from build123d import *

# Parameters (mm, degrees)
F1_DEPTH      = 12.7
F1_DEPTH_BACK = 12.7
F0_W          = 371.475
F0_H          = 622.3
F2_DEPTH      = 9.398
F2_DEPTH_BACK = 9.398
F3_W          = 371.475
F3_H          = 12.7
F4_DEPTH      = 12.7


# Not quite as in the source:
# - a feature names something its author has since deleted; it is built from what else it names


with BuildPart() as f1:
    # F0 (on Front) → F1 (new body, two sides)
    with BuildSketch(Plane.XZ) as f1_sk:
        Polygon((263.0418609804, 506.0493900317), (634.5168609804, 506.0493900317), (653.5668609804, 525.0993900317), (243.9918609804, 525.0993900317), align=None)
        Polygon((653.5668609804, 525.0993900317), (634.5168609804, 506.0493900317), (634.5168609804, -116.2506099683), (653.5668609804, -135.3006099683), align=None)
        Polygon((653.5668609804, -135.3006099683), (634.5168609804, -116.2506099683), (263.0418609804, -116.2506099683), (243.9918609804, -135.3006099683), align=None)
        Polygon((263.0418609804, -116.2506099683), (263.0418609804, 506.0493900317), (243.9918609804, 525.0993900317), (243.9918609804, -135.3006099683), align=None)
    extrude(amount=-F1_DEPTH)
    extrude(f1_sk.sketch, amount=F1_DEPTH_BACK)

    # F0 (on Front) → F2 (join, two sides)
    with BuildSketch(Plane.XZ) as f2_sk:
        Polygon((653.5668609804, 525.0993900317), (634.5168609804, 506.0493900317), (634.5168609804, -116.2506099683), (653.5668609804, -135.3006099683), align=None)
        Polygon((263.0418609804, 506.0493900317), (634.5168609804, 506.0493900317), (653.5668609804, 525.0993900317), (243.9918609804, 525.0993900317), align=None)
        Polygon((653.5668609804, -135.3006099683), (634.5168609804, -116.2506099683), (263.0418609804, -116.2506099683), (243.9918609804, -135.3006099683), align=None)
        with Locations((448.7793609804, 194.8993900317)):
            Rectangle(F0_W, F0_H)
        Polygon((263.0418609804, -116.2506099683), (263.0418609804, 506.0493900317), (243.9918609804, 525.0993900317), (243.9918609804, -135.3006099683), align=None)
    extrude(amount=-F2_DEPTH)
    extrude(f2_sk.sketch, amount=F2_DEPTH_BACK)

    # F3 (on face) → F4 (cut)
    with BuildSketch(Plane.XZ):
        Polygon((455.1293609804, 105.9993900317), (455.1293609804, 384.1293900317), (634.5168609804, 384.1293900317), (634.5168609804, 396.8293900317), (263.0418609804, 396.8293900317), (263.0418609804, 384.1293900317), (442.4293609804, 384.1293900317), (442.4293609804, 105.9993900317), (263.0418609804, 105.9993900317), (263.0418609804, 93.2993900317), (634.5168609804, 93.2993900317), (634.5168609804, 105.9993900317), align=None)
        with Locations((448.7793609804, -8.3006099683)):
            Rectangle(F3_W, F3_H)
    extrude(amount=F4_DEPTH, mode=Mode.SUBTRACT)


solid = f1.part
Part model, mm, in its own coordinate system. A direction names the side the tool comes from. Coordinates: 2 decimals unless noted, no trailing zeros. Loops run counter-clockwise (first coordinate to the right, second up) from the corner with the lowest first, then second, coordinate; pieces in that order, holes last. Notation, with made-up numbers: M 1,9.5 L 32,9.5 A20 cw 32,43.5 Z; hole C 24.5,1 d3. An arc over 180 degrees is marked long. Use a Markdown table: item, result. Add a question column.
Q1. Mould opens along Z. For faces 4 (the flat face through (634.517, -11, 173)), 5 (the flat face through (251, -12.7, 196)), 6 (the flat face through (446, 0, -135.301)) say: +Z half, -Z half, draft (parallel to the pull), parting line (faces both ways), or undercut.
Q2. Cut at B-B (x = 592.5). Write the cut outline in (y, z).
Q3. Pin check, flat tip, straight feed: P1, Ø1, axis at x = 572, z = 402.5, coming from the -Y side. Stop position of the tip, or through.
Q4. Cut at C-C (y = -5). Write the cut outline in (x, z), and give its area (3 significant figures).
Q5. Cut at A-A (z = 354). Write the cut outline in (x, y), and give its area (3 significant figures).
Q6. Cut at D-D (z = -33). Write the cut outline in (x, y).
Q7. Probe L1, parallel to Z at x = 541, y = -3.5; L2, parallel to X at y = 11, z = -15; L3, parallel to Z at x = 467, y = 10.75. List the from-to ranges inside material, lowest first.
Q8. Which spindle directions (+Z, -Z, +X, -X, +Y, -Y) get a long thin tool onto all of the face, cutting with end or side? Do faces 1 (the flat face through (446, 9.398, 199)), 2 (the flat face through (446, -9.398, -65)), 3 (the flat face through (452, 0, 525.099)). Say none if no direction does.
Worked out:
| question | item | result |
|---|---|---|
| 1 | face 4 | undercut |
| 1 | face 5 | draft |
| 1 | face 6 | -Z half |
| 2 | outline | M -12.7,-135.3 L 12.7,-135.3 L 12.7,-116.25 L 9.4,-116.25 L 9.4,506.05 L 12.7,506.05 L 12.7,525.1 L -12.7,525.1 L -12.7,506.05 L -9.4,506.05 L -9.4,396.83 L 0,396.83 L 0,384.13 L -9.4,384.13 L -9.4,106 L 0,106 L 0,93.3 L -9.4,93.3 L -9.4,-1.95 L 0,-1.95 L 0,-14.65 L -9.4,-14.65 L -9.4,-116.25 L -12.7,-116.25 Z |
| 3 | P1 | stops at y = -9.4 |
| 4 | outline | M 243.99,-135.3 L 653.57,-135.3 L 653.57,525.1 L 243.99,525.1 Z; hole M 263.04,-14.65 L 634.52,-14.65 L 634.52,-1.95 L 263.04,-1.95 Z; hole M 263.04,93.3 L 634.52,93.3 L 634.52,106 L 455.13,106 L 455.13,384.13 L 634.52,384.13 L 634.52,396.83 L 263.04,396.83 L 263.04,384.13 L 442.43,384.13 L 442.43,106 L 263.04,106 Z |
| 4 | area | 253,000 mm2 |
| 5 | outline | M 243.99,-12.7 L 263.04,-12.7 L 263.04,-9.4 L 442.43,-9.4 L 442.43,0 L 455.13,0 L 455.13,-9.4 L 634.52,-9.4 L 634.52,-12.7 L 653.57,-12.7 L 653.57,12.7 L 634.52,12.7 L 634.52,9.4 L 263.04,9.4 L 263.04,12.7 L 243.99,12.7 Z |
| 5 | area | 7,830 mm2 |
| 6 | outline | M 243.99,-12.7 L 263.04,-12.7 L 263.04,-9.4 L 634.52,-9.4 L 634.52,-12.7 L 653.57,-12.7 L 653.57,12.7 L 634.52,12.7 L 634.52,9.4 L 263.04,9.4 L 263.04,12.7 L 243.99,12.7 Z |
| 7 | L1 | z = -135.3 to -14.65, -1.95 to 93.3, 106 to 384.13, 396.83 to 525.1 |
| 7 | L2 | x = 243.99 to 263.04, 634.52 to 653.57 |
| 7 | L3 | z = -135.3 to -116.25, 506.05 to 525.1 |
| 8 | face 1 | +Y |
| 8 | face 2 | -Y |
| 8 | face 3 | +Z, +X, -X, +Y, -Y |
